Could you check a few things on this model? Use its own coordinates, in mm. A direction names the side the tool comes from. Give positions to 0.01 mm unless a question says otherwise; leave off trailing zeros. Loops run counter-clockwise (first coordinate to the right, second up) from the corner with the lowest first, then second, coordinate; pieces in that order, holes last. Notation, with made-up numbers: (-4.75, 82.5) -> (12.25, 82.5) arc R10 ccw to (12.25, 88.5) -> close; hole circle Ø5 at (72.25, 51). An arc over 180 degrees is marked (long way). Write item = value, one per line. Start each with the question number.
1) I need wall thicknesses on probe 1 along Z at (x, y) = (0.75, -1); probe 2 along Z at (x, y) = (0, -3.5); probe 3 along Y at (x, z) = (1.25, 2.25). Which ranges of each line are inside material? Lowest first, please. Write a range as from..to.
2) I want a section at B-B (z = 4). List the corners of the cut face in (x, y) for me, and give its area (3 significant figures).
3) If we mould it in two halves opening along Y, with no side actions, what happens to faces 1 (the face through (2, -2, 5)), 2 (the face through (-0.867, -3.905, 2.472)), 3 (the face through (1.014, -1.724, 1.58))? For each: +Y half, -Y half, draft (parallel to the pull), parting line (faces both ways), or undercut.
4) On a 3-axis mill with a long thin cutter (end or side, diameter ignored), from which of +Z, -Z, +X, -X, +Y, -Y can I reach the whole of each face in a straight line? I mean faces 4 (the face through (-0.54, -2.44, 8.25)), 5 (the face through (-0.8, -2.3, 0)), 6 (the face through (-1.01, 1.79, 0.06)). Say none if no direction works.
5) I'm going to push a flat-ended pin straight in: pin 1 Ø1.2 at (x, y) = (0, 0) entering from -Z. Where does the tip first touch, or does it pass through?
6) I want a section at A-A (y = 0). List the corners of the cut face in (x, z) for me.
7) I want a section at C-C (z = 6.75). List the corners of the cut face in (x, y) for me.
from build123d import *

# Parameters (mm, degrees)
ESBO_O1_R                = 4
RESSALTO_EXTRUS_O1_DEPTH = 5
ESBO_O2_R                = 2.5
RESSALTO_EXTRUS_O2_DEPTH = 7
CORTE_EXTRUS_O1_DEPTH    = 3
FILETE1_R                = 0.5
FILETE2_R                = 0.2
CHANFRO2_SIZE            = 0.4


with BuildPart() as part:
    # Esboço1 → Ressalto-extrusão1 (new body)
    with BuildSketch(Plane.XY):
        Circle(ESBO_O1_R)
    extrude(amount=RESSALTO_EXTRUS_O1_DEPTH)

    # Esboço2 → Ressalto-extrusão2 (add)
    with BuildSketch(Plane.XY.offset(5)):
        Circle(ESBO_O2_R)
    extrude(amount=RESSALTO_EXTRUS_O2_DEPTH)

    # Esboço3 → Corte-extrusão1 (cut)
    with BuildSketch(Plane(origin=(0, 0, 0), x_dir=(-1, 0, 0), z_dir=(0, 0, -1))):
        Polygon((0, 2.309401077), (-2, 1.154700538), (-2, -1.154700538), (0, -2.309401077), (2, -1.154700538), (2, 1.154700538), align=None)
    extrude(amount=-CORTE_EXTRUS_O1_DEPTH, mode=Mode.SUBTRACT)

    # Filete1
    filete1_edges = [part.edges().sort_by_distance(p)[0] for p in [
        (-4, 0, 0),
        (-4, 0, 5),
    ]]
    fillet(filete1_edges, radius=FILETE1_R)

    # Filete2
    filete2_edges = [part.edges().sort_by_distance(p)[0] for p in [
        (-1, 1.732050808, 0),
        (1, 1.732050808, 0),
        (2, 0, 0),
        (1, -1.732050808, 0),
        (-1, -1.732050808, 0),
        (-2, 0, 0),
    ]]
    fillet(filete2_edges, radius=FILETE2_R)

    # Chanfro2
    chanfro2_edges = [part.edges().sort_by_distance(p)[0] for p in [
        (-2.5, 0, 12),
    ]]
    chamfer(chanfro2_edges, length=CHANFRO2_SIZE)


solid = part.part
Answer list:
q1.probe_1 = 3..12
q1.probe_2 = 0..5
q1.probe_3 = -3.8..-1.59, 1.59..3.8
q2.outline = circle Ø8 at (0, 0)
q2.area = 50.3 mm^2
q3.face_1 = draft
q3.face_2 = parting line
q3.face_3 = undercut
q4.face_4 = +Z
q4.face_5 = -Z, +X, -X, +Y, -Y
q4.face_6 = -Z
q5.pin_1 = 3
q6.outline = (-4, 0.5) arc R0.5 ccw to (-3.5, 0) -> (-2.2, 0) arc R0.2 ccw to (-2, 0.2) -> (-2, 3) -> (2, 3) -> (2, 0.2) arc R0.2 ccw to (2.2, 0) -> (3.5, 0) arc R0.5 ccw to (4, 0.5) -> (4, 4.5) arc R0.5 ccw to (3.5, 5) -> (2.5, 5) -> (2.5, 11.6) -> (2.1, 12) -> (-2.1, 12) -> (-2.5, 11.6) -> (-2.5, 5) -> (-3.5, 5) arc R0.5 ccw to (-4, 4.5) -> close
q7.outline = circle Ø5 at (0, 0)
